Design review of the part built by this model. Coordinates are the model's own, in mm. A direction names the side the tool comes from. Coordinates: 2 decimals unless noted, no trailing zeros. Loops run counter-clockwise (first coordinate to the right, second up) from the corner with the lowest first, then second, coordinate; pieces in that order, holes last. Notation, with made-up numbers: (-31.75, 14) -> (20.25, 14) arc R15 cw to (20.25, 23) -> close; hole circle Ø10 at (0.25, 24). An arc over 180 degrees is marked (long way). Answer in a Markdown table with one row per item.
```python
from build123d import *

# Parameters (mm, degrees)
BOSS_EXTRUDE1_DEPTH            = 15.24
CUT_EXTRUDE1_DEPTH             = 97.554341556
CBORE_FOR_M3_SBHCS2_AT_2_COUNT = 2
CBORE_FOR_M3_SBHCS2_AT_2_PITCH = 41.005
CBORE_FOR_M3_SBHCS2_AT_3_COUNT = 2
CBORE_FOR_M3_SBHCS2_AT_3_PITCH = 61.832422118
CBORE_FOR_M3_SBHCS2_AT_4_COUNT = 2
CBORE_FOR_M3_SBHCS2_AT_4_PITCH = 46.28
SKETCH16_R                     = 3.35
CUT_EXTRUDE2_DEPTH             = 98.872548965


with BuildPart() as part:
    # Sketch2 → Boss-Extrude1 (new body)
    with BuildSketch(Plane(origin=(0, 0, 0), x_dir=(1, 0, 0), z_dir=(0, 1, 0))):
        with BuildLine():
            Line((81.8747525, 30.528055776), (12.1947525, 30.528055776))
            ThreePointArc((12.1947525, 30.528055776), (5.010547603, 27.552260673), (2.0347525, 20.368055776))
            Line((2.0347525, 20.368055776), (2.0347525, -21.311944224))
            ThreePointArc((2.0347525, -21.311944224), (5.010547603, -28.496149121), (12.1947525, -31.471944224))
            Line((12.1947525, -31.471944224), (81.8747525, -31.471944224))
            ThreePointArc((81.8747525, -31.471944224), (89.058957397, -28.496149121), (92.0347525, -21.311944224))
            Line((92.0347525, -21.311944224), (92.0347525, 20.368055776))
            ThreePointArc((92.0347525, 20.368055776), (89.058957397, 27.552260673), (81.8747525, 30.528055776))
        make_face()
        with BuildLine():
            Line((16.5547525, 17.943055776), (77.5147525, 17.943055776))
            ThreePointArc((77.5147525, 17.943055776), (81.106854948, 16.455158224), (82.5947525, 12.863055776))
            Line((82.5947525, 12.863055776), (82.5947525, -13.806944224))
            ThreePointArc((82.5947525, -13.806944224), (81.106854948, -17.399046672), (77.5147525, -18.886944224))
            Line((77.5147525, -18.886944224), (16.5547525, -18.886944224))
            ThreePointArc((16.5547525, -18.886944224), (12.962650051, -17.399046672), (11.4747525, -13.806944224))
            Line((11.4747525, -13.806944224), (11.4747525, 12.863055776))
            ThreePointArc((11.4747525, 12.863055776), (12.962650051, 16.455158224), (16.5547525, 17.943055776))
        make_face(mode=Mode.SUBTRACT)
    extrude(amount=BOSS_EXTRUDE1_DEPTH)

    # Sketch3 → Cut-Extrude1 (cut, through all)
    with BuildSketch(Plane.ZY.offset(-2.0347525)):
        Polygon((21.311944224, 15.24), (-20.368055776, 15.24), (-30.528055776, 15.24), (31.471944224, 5.4201647), (31.471944224, 15.24), align=None)
    extrude(amount=-CUT_EXTRUDE1_DEPTH, mode=Mode.SUBTRACT)

    # Sketch15 → CBORE for M3 SBHCS2 (revolve, cut)
    with BuildSketch(Plane(origin=(67.5372525, 4.37, 23.611944224), x_dir=(0, 0, 1), z_dir=(1, 0, 0))):
        Polygon((0, 0), (0, 4.37), (1.8, 4.37), (1.8, 1.65), (3.35, 1.65), (3.35, 0), align=None)
    cbore_for_m3_sbhcs2 = revolve(axis=Axis((67.5372525, 10.72, 23.611944224), (0, -1, 0)), mode=Mode.SUBTRACT)

    # CBORE for M3 SBHCS2 at 2: CBORE for M3 SBHCS2 ×2
    with Locations(*[(-i * CBORE_FOR_M3_SBHCS2_AT_2_PITCH, 0, 0) for i in range(1, CBORE_FOR_M3_SBHCS2_AT_2_COUNT)]):
        add(cbore_for_m3_sbhcs2, mode=Mode.SUBTRACT)

    # CBORE for M3 SBHCS2 at 3: CBORE for M3 SBHCS2 ×2
    with Locations(*[Vector(-0.6631634116100382, 0, -0.7484746418561787) * (i * CBORE_FOR_M3_SBHCS2_AT_3_PITCH) for i in range(1, CBORE_FOR_M3_SBHCS2_AT_3_COUNT)]):
        add(cbore_for_m3_sbhcs2, mode=Mode.SUBTRACT)

    # CBORE for M3 SBHCS2 at 4: CBORE for M3 SBHCS2 ×2
    with Locations(*[(0, 0, -i * CBORE_FOR_M3_SBHCS2_AT_4_PITCH) for i in range(1, CBORE_FOR_M3_SBHCS2_AT_4_COUNT)]):
        add(cbore_for_m3_sbhcs2, mode=Mode.SUBTRACT)

    # Sketch16 → Cut-Extrude2 (cut, through all)
    with BuildSketch(Plane(origin=(0, 4.37, 0), x_dir=(-1, 0, 0), z_dir=(0, -1, 0))):
        with Locations(Location((-67.5372525, -23.611944224, 0), (0, 0, 270))):
            Circle(SKETCH16_R)
        with Locations(Location((-26.5322525, -23.611944224, 0), (0, 0, 270))):
            Circle(SKETCH16_R)
        with Locations(Location((-67.5372525, 22.668055776, 0), (0, 0, 270))):
            Circle(SKETCH16_R)
        with Locations(Location((-26.5322525, 22.668055776, 0), (0, 0, 270))):
            Circle(SKETCH16_R)
    extrude(amount=-CUT_EXTRUDE2_DEPTH, mode=Mode.SUBTRACT)


solid = part.part
```
(1) Take a section at D-D on z = -23.5. Give the boundary of the cut face in (x, y), and give its area (3 significant figures).
Evaluation:
| item | result |
|---|---|
| outline | (2.53, 0) -> (24.94, 0) -> (24.94, 2.72) -> (23.29, 2.72) -> (23.29, 14.13) -> (2.53, 14.13) -> close; (28.13, 0) -> (65.94, 0) -> (65.94, 2.72) -> (64.29, 2.72) -> (64.29, 14.13) -> (29.78, 14.13) -> (29.78, 2.72) -> (28.13, 2.72) -> close; (69.13, 0) -> (91.54, 0) -> (91.54, 14.13) -> (70.78, 14.13) -> (70.78, 2.72) -> (69.13, 2.72) -> close |
| area | 1,090 mm² |
(2) Tool access review of faces 1 (the flat face through (48, 8, -30.528)), 2 (the cylindrical face through (13.002, 4.051, 17.438)), 3 (the flat face through (28, 2.72, 22)): name each direction out of +Z, -Z, +X, -X, +Y, -Y from which nothing blocks a thin tool from reaching the whole face with its end or side.
Evaluation:
| item | result |
|---|---|
| face 1 | -Z, +X, -X, +Y, -Y |
| face 2 | +Y, -Y |
| face 3 | +Y |
(3) Take a section at B-B on z = -15. Give the boundary of the cut face in (x, y), and give its area (3 significant figures).
Evaluation:
| item | result |
|---|---|
| outline | (2.03, 0) -> (11.95, 0) -> (11.95, 12.78) -> (2.03, 12.78) -> close; (82.12, 0) -> (92.03, 0) -> (92.03, 12.78) -> (82.12, 12.78) -> close |
| area | 253 mm² |
(4) Draft analysis for pull direction Z (two halves, no side actions). For faces 4 (the cylindrical face through (88.98, 2.684, 28.575)), 5 (the cylindrical face through (81.07, 6.53, -16.49)), 6 (the flat face through (46, 0, -21)), state which applies: pulls with the +Z half, pulls with the -Z half, needs draft (parallel to the pull), parting line crosses it, or undercut.
Evaluation:
| item | result |
|---|---|
| face 4 | pulls with the +Z half |
| face 5 | undercut |
| face 6 | needs draft |
(5) For pin 1 (4 mm diameter, centred on x = 26.53, z = -22.67, fed in from +Y); pin 2 (3 mm diameter, centred on x = 67.54, z = -22.67, fed in from +Y); pin 3 (8 mm diameter, centred on x = 32.5, z = 18, fed in from +Y); pin 4 (12 mm diameter, centred on x = 75.5, z = -23, fed in from +Y), all flat-tipped, find the tip position at first contact; note any pin that passes through.
Evaluation:
| item | result |
|---|---|
| pin 1 | stops at y = 2.72 |
| pin 2 | passes through |
| pin 3 | stops at y = 7.41 |
| pin 4 | stops at y = 15 |
(6) Take a section at A-A on x = 57.5. Give the boundary of the cut face in (y, z), and give its area (3 significant figures).
Evaluation:
| item | result |
|---|---|
| outline | (0, -30.53) -> (15.24, -30.53) -> (13.25, -17.94) -> (0, -17.94) -> close; (0, 18.89) -> (7.41, 18.89) -> (5.42, 31.47) -> (0, 31.47) -> close |
| area | 260 mm² |
(7) To check wall thickness, follow probe 1 along X at (y, z) = (6, 7); probe 2 along Z at (x, y) = (63.5, 4); probe 3 along Z at (x, y) = (62.5, 12.75). State the ranges of each line that lie inside material, in increasing order.
Evaluation:
| item | result |
|---|---|
| probe 1 | x = 2.03 to 11.47, 82.59 to 92.03 |
| probe 2 | z = -30.53 to -17.94, 18.89 to 31.47 |
| probe 3 | z = -30.53 to -17.94 |
(8) Take a section at C-C on y = 10.5. Give the boundary of the cut face in (x, z), and give its area (3 significant figures).
Evaluation:
| item | result |
|---|---|
| outline | (2.03, -20.37) arc R10.16 ccw to (12.19, -30.53) -> (81.87, -30.53) arc R10.16 ccw to (92.03, -20.37) -> (92.03, -0.6) -> (82.59, -0.6) -> (82.59, -12.86) arc R5.08 cw to (77.51, -17.94) -> (16.55, -17.94) arc R5.08 cw to (11.47, -12.86) -> (11.47, -0.6) -> (2.03, -0.6) -> close; hole circle Ø6.7 at (26.53, -22.67); hole circle Ø6.7 at (67.54, -22.67) |
| area | 1,360 mm² |
